Could you check a few things on this drawing? It's one solid part, dimensions in mm from its lowest x, y, z. A direction names the side the tool comes from. Give positions to 0.01 mm unless a question says otherwise; leave off trailing zeros. Order: outer loops, then holes, each group sorted by start corner. A loop starts at its lowest first (then second) coordinate and runs counter-clockwise, first axis right, second up. Notation, with made-up numbers: (13.5, 81) -> (41.5, 81) arc R24 cw to (41.5, 118) -> close; hole circle Ø5 at (-18.5, 14). An arc over 180 degrees is marked (long way). Write each question's results on one line, items separated by ' | '.
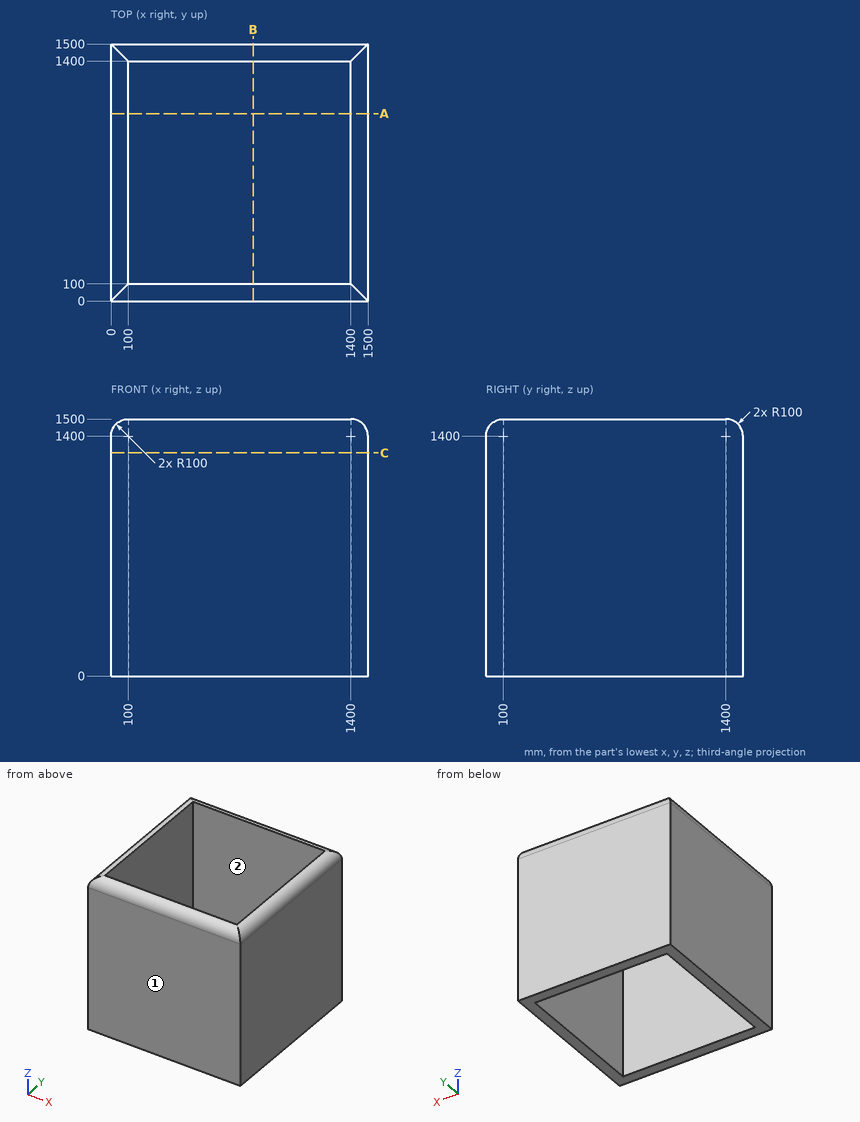
Q1. For the marked faces 1 and 2, which set-ups out of +Z, -Z, +X, -X, +Y, -Y let a thin tool reach every point of the face, with its end or its side?
Here are the results:
face 1: +Z, -Z, +X, -X, -Y | face 2: +Z, -Z
Q2. Suppose I cut it at A-A on y = 1093. Please give me the cut outline in (x, z), and give its area (3 significant figures).
Here are the results:
outline: (0, 0) -> (100, 0) -> (100, 1500) arc R100 ccw to (0, 1400) -> close; (1400, 0) -> (1500, 0) -> (1500, 1400) arc R100 ccw to (1400, 1500) -> close | area: 296,000 mm²
Q3. I need wall thicknesses on line 1 along X through (y, z) = (1270.5, 963); line 2 along X through (y, z) = (134.5, 1417). Which ranges of each line are inside material? Lowest first, please.
Here are the results:
line 1: x = 0 to 100, 1400 to 1500 | line 2: x = 1.46 to 100, 1400 to 1498.54
Q4. Suppose I cut it at C-C on z = 1302.5. Please give me the cut outline in (x, y), and give its area (3 significant figures).
Here are the results:
outline: (0, 0) -> (1500, 0) -> (1500, 1500) -> (0, 1500) -> close; hole (100, 100) -> (1400, 100) -> (1400, 1400) -> (100, 1400) -> close | area: 560,000 mm²
